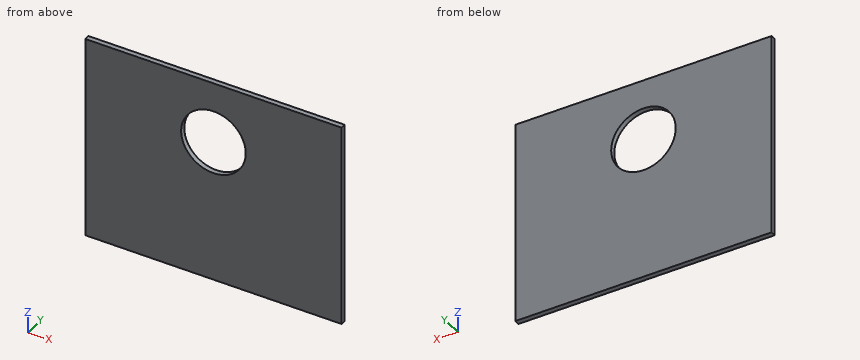
from build123d import *

# Parameters (mm, degrees)
SKETCH1_W           = 500
SKETCH1_H           = 400
BOSS_EXTRUDE1_DEPTH = 10
SKETCH2_R           = 63
CUT_EXTRUDE1_DEPTH  = 20


with BuildPart() as part:
    # Sketch1 → Boss-Extrude1 (new body)
    with BuildSketch(Plane(origin=(0, 0, 0), x_dir=(1, 0, 0), z_dir=(0, 1, 0))):
        Rectangle(SKETCH1_W, SKETCH1_H)
    extrude(amount=-BOSS_EXTRUDE1_DEPTH)

    # Sketch2 → Cut-Extrude1 (cut)
    with BuildSketch(Plane(origin=(0, 0, 0), x_dir=(1, 0, 0), z_dir=(0, 1, 0))):
        with Locations((0, -80)):
            Circle(SKETCH2_R)
    extrude(amount=-CUT_EXTRUDE1_DEPTH, mode=Mode.SUBTRACT)


solid = part.part
Design review of the part built by this model. Coordinates are the model's own, in mm. Round coordinates to 2 decimals unless told otherwise and drop trailing zeros. Write each loop counter-clockwise with the first axis right and the second up, starting at its lowest first coordinate (ties: lowest second). Pieces come first, ordered by that corner, then holes.
Item 1: Consider section A-A on x = 0. Give the boundary of the cut face in (y, z), and give its area (3 significant figures).
Item 2: Consider section C-C on z = 80. Give the boundary of the cut face in (x, y).
Item 3: Wall thickness on L1, parallel to X at y = -4, z = 80; L2, parallel to Z at x = 0, y = -5.25; L3, parallel to X at y = -2.25, z = 133: over which ranges is each line inside the solid? List them lowest first.
Item 4: Consider section B-B on y = -3. Give the boundary of the cut face in (x, z), and give its area (3 significant figures).
Check values:
1. outline: (-10, -200) - (0, -200) - (0, 17) - (-10, 17) - close; (-10, 143) - (0, 143) - (0, 200) - (-10, 200) - close
1. area: 2,740 mm2
2. outline: (-250, -10) - (-63, -10) - (-63, 0) - (-250, 0) - close; (63, -10) - (250, -10) - (250, 0) - (63, 0) - close
3. L1: x = -250 to -63, 63 to 250
3. L2: z = -200 to 17, 143 to 200
3. L3: x = -250 to -34.06, 34.06 to 250
4. outline: (-250, -200) - (250, -200) - (250, 200) - (-250, 200) - close; hole circle Ø126 at (0, 80)
4. area: 188,000 mm2
